```python
from build123d import *

# Parameters (mm, degrees)
SKETCH1_R           = 28.575
SKETCH1_R_2         = 2.5908
BOSS_EXTRUDE1_DEPTH = 6.35
SKETCH2_R           = 12.192
BOSS_EXTRUDE2_DEPTH = 19.05
CUT_EXTRUDE1_DEPTH  = 26.4


with BuildPart() as part:
    # Sketch1 → Boss-Extrude1 (new body)
    with BuildSketch(Plane.XY):
        Circle(SKETCH1_R)
        with Locations((0, 23.8125)):
            Circle(SKETCH1_R_2, mode=Mode.SUBTRACT)
        with Locations((20.622229928, 11.90625)):
            Circle(SKETCH1_R_2, mode=Mode.SUBTRACT)
        with Locations((20.622229928, -11.90625)):
            Circle(SKETCH1_R_2, mode=Mode.SUBTRACT)
        with Locations((0, -23.8125)):
            Circle(SKETCH1_R_2, mode=Mode.SUBTRACT)
        with Locations((-20.622229928, -11.90625)):
            Circle(SKETCH1_R_2, mode=Mode.SUBTRACT)
        with Locations((-20.622229928, 11.90625)):
            Circle(SKETCH1_R_2, mode=Mode.SUBTRACT)
    extrude(amount=BOSS_EXTRUDE1_DEPTH)

    # Sketch2 → Boss-Extrude2 (add)
    with BuildSketch(Plane(origin=(0, 0, 0), x_dir=(-1, 0, 0), z_dir=(0, 0, -1))):
        Circle(SKETCH2_R)
    extrude(amount=BOSS_EXTRUDE2_DEPTH)

    # Sketch3 → Cut-Extrude1 (cut, through all)
    with BuildSketch(Plane.XY.offset(6.35)):
        Polygon((6.42148496, -3.688971027), (6.405485103, 3.716683592), (-0.015999857, 7.405654619), (-6.42148496, 3.688971027), (-6.405485103, -3.716683592), (0.015999857, -7.405654619), align=None)
    extrude(amount=-CUT_EXTRUDE1_DEPTH, mode=Mode.SUBTRACT)


solid = part.part
```
Input: part model. Units: mm. Frame: model coordinates. A direction names the side the tool comes from. Round coordinates to 2 decimals unless told otherwise and drop trailing zeros. Loops run counter-clockwise (first coordinate to the right, second up) from the corner with the lowest first, then second, coordinate; pieces in that order, holes last. Notation, with made-up numbers: M 33,-27.75 L 69,-27.75 A18 cw 69,7.25 Z; hole C -0.5,68 d3. An arc over 180 degrees is marked long. Answer in a Markdown table with one row per item. Add a question column.
1. Section A-A (z = -10.5). Output: boundary loops of the cut face in (x, y), and give its area (3 significant figures).
2. Section B-B (y = 0). Output: boundary loops of the cut face in (x, z) (3 decimals).
3. Ray query, probe 1 along Y at (x, z) = (0, 4) (3 decimals); probe 2 along X at (y, z) = (-12, 0.25); probe 3 along Z at (x, y) = (18.5, -6). Return the intervals inside material, ascending.
4. Mould query, pull axis X, two halves, no side actions, for faces 3 (the face through (-19.23, -9.72, 3.13)), 4 (the face through (12, -6, 0)), 5 (the face through (1.587, 12.088, -9.392)). Classes: released by +X, released by -X, zero draft, split by the parting line, or undercut.
5. Section C-C (x = 5). Output: boundary loops of the cut face in (y, z).
6. Set-up query: faces 1 (the face through (3.24, 5.535, -6.172)), 2 (the face through (-5, -5, -19.05)). Return all of +Z, -Z, +X, -X, +Y, -Y with unobstructed straight access to the full face (end or side cutting, diameter ignored); none if empty.
7. Contact query for flat-ended pins moving along their axis: pin 1 (6 mm diameter, centred on x = 20.62, y = 11.91, fed in from -Z); pin 2 (5 mm diameter, centred on x = -15, z = 1, fed in from -Y); pin 3 (5 mm diameter, centred on x = 3.5, z = 0, fed in from +Y); pin 4 (4 mm diameter, centred on x = 20.62, y = -11.91, fed in from +Z). Output: stop coordinate, or through.
8. Section D-D (x = 22.5). Output: boundary loops of the cut face in (y, z), and give its area (3 significant figures).
Values follow:
| question | item | result |
|---|---|---|
| 1 | outline | C 0,0 d24.38; hole M -6.42,3.69 L -6.41,-3.72 L 0.02,-7.41 L 6.42,-3.69 L 6.41,3.72 L -0.02,7.41 Z |
| 1 | area | 324 mm^2 |
| 2 | outline | M -28.575,0 L -12.192,0 L -12.192,-19.05 L -6.414,-19.05 L -6.414,6.35 L -28.575,6.35 Z; M 6.414,-19.05 L 12.192,-19.05 L 12.192,0 L 28.575,0 L 28.575,6.35 L 6.414,6.35 Z |
| 3 | probe 1 | -28.575 to -26.403, -21.222 to -7.396, 7.396 to 21.222, 26.403 to 28.575 |
| 3 | probe 2 | -25.93 to -23.21, -18.03 to 18.03, 23.21 to 25.93 |
| 3 | probe 3 | 0 to 6.35 |
| 4 | face 3 | undercut |
| 4 | face 4 | zero draft |
| 4 | face 5 | split by the parting line |
| 5 | outline | M -28.13,0 L -11.12,0 L -11.12,-19.05 L -4.51,-19.05 L -4.51,6.35 L -28.13,6.35 Z; M 4.52,-19.05 L 11.12,-19.05 L 11.12,0 L 28.13,0 L 28.13,6.35 L 4.52,6.35 Z |
| 6 | face 1 | +Z, -Z |
| 6 | face 2 | -Z, +X, -X, +Y, -Y |
| 7 | pin 1 | z = 0 |
| 7 | pin 2 | y = -25.7 |
| 7 | pin 3 | y = 28.56 |
| 7 | pin 4 | through |
| 8 | outline | M -17.61,0 L -13.69,0 L -13.69,6.35 L -17.61,6.35 Z; M -10.12,0 L 10.12,0 L 10.12,6.35 L -10.12,6.35 Z; M 13.69,0 L 17.61,0 L 17.61,6.35 L 13.69,6.35 Z |
| 8 | area | 178 mm^2 |
